Geometry: final body of the model. Coordinates: model frame, mm. A direction names the side the tool comes from. Round coordinates to 2 decimals unless told otherwise and drop trailing zeros. Order: outer loops, then holes, each group sorted by start corner. A loop starts at its lowest first (then second) coordinate and runs counter-clockwise, first axis right, second up. Notation, with made-up numbers: M 45,33.5 L 67,33.5 A15 ccw 67,62.5 Z; hole C 73.5,-35.75 d3. An arc over 180 degrees is marked long. Put each result on its own line as item: value. Start each with the question number.
1) Access query for faces 1 (the flat face through (-8.38, 15.21, 34.31)), 2 (the flat face through (35.002, 15.21, 4.747)), 3 (the flat face through (-31.107, 15.21, 16.734)), 4 (the flat face through (-21.61, 15.21, 27.94)), 5 (the flat face through (6.22, 15.21, -34.64)). Directions: +Z, -Z, +X, -X, +Y, -Y. A direction counts if a zero-diameter tool reaches every point of the face in a straight line with its end or side. Return the directions, or none.
2) First-contact query: P1, Ø1.5, axis at x = 13.5, y = 11, coming from the +Z side; P2, Ø5, axis at x = -3, z = -16, coming from the +Y side; P3, Ø3, axis at y = 9.5, z = 29.5, coming from the +X side; P4, Ø3, axis at y = 22, z = 22.5, coming from the -X side. Flat tips, straight axial feed; report the tip coordinate or a pass-through.
3) Section B-B, the plane z = -10. Return loops of the section in (x, y), then the cut area to 3 significant figures.
4) Draft query along Z for faces 6 (the flat face through (8.5, 0, 18.3)), 7 (the cylindrical face through (26.73, 15.21, 29.76)), 8 (the flat face through (-13.39, 15.21, -32.686)), 9 (the flat face through (33.907, 15.21, -9.9)). Return one class per face: pulls with the +Z half, pulls with the -Z half, needs draft (parallel to the pull), parting line crosses it, or undercut.
5) Section C-C, the plane x = -24.5. Return loops of the section in (y, z), then the cut area to 3 significant figures.
6) Material intervals for probe 1 along Z at (x, y) = (28, 8.5); probe 2 along Z at (x, y) = (28.5, 2.5); probe 3 along Z at (x, y) = (-33.5, 25.5), sorted ascending. Write a range as [from, to].
7) Section A-A, the plane x = 6. Return loops of the section in (y, z).
from build123d import *

# Parameters (mm, degrees)
SKETCH_2_W               = 20
SKETCH_2_H               = 30
CUT_EXTRUDE_1_DEPTH      = 65.031242374
PATTERN_CIRCULAR_2_COUNT = 15


with BuildPart() as part:
    # 草图2 → 旋转1 (revolve)
    with BuildSketch(Plane.XY, mode=Mode.PRIVATE) as revolve_1_sk:
        with Locations((-30, 15)):
            Rectangle(SKETCH_2_W, SKETCH_2_H)
    revolve(revolve_1_sk.sketch.rotate(Axis((0, 0, 0), (0, 1, 0)), 270), axis=Axis((0, 0, 0), (0, 1, 0)))

    # 草图3 → 切除-拉伸1 (cut, through all)
    with BuildSketch(Plane(origin=(0, 30, 0), x_dir=(1, 0, 0), z_dir=(0, 1, 0))):
        Polygon((-30.66106403, 0), (-39.66106403, 5.196152423), (-48.66106403, 0), (-39.66106403, -5.196152423), align=None)
    cut_extrude_1 = extrude(amount=-CUT_EXTRUDE_1_DEPTH, mode=Mode.SUBTRACT)

    # 阵列(圆周)2: 切除-拉伸1 ×15 about axis
    pattern_circular_2_axis = Axis((0, 0, 0), (0, 1, 0))
    for i in range(1, PATTERN_CIRCULAR_2_COUNT):
        add(cut_extrude_1.rotate(pattern_circular_2_axis, i * 360 / PATTERN_CIRCULAR_2_COUNT), mode=Mode.SUBTRACT)


solid = part.part
Result sheet:
1. face 1: +Z, +Y, -Y
1. face 2: +X, +Y, -Y
1. face 3: -X, +Y, -Y
1. face 4: +Y, -Y
1. face 5: -Z, +Y, -Y
2. P1: stops at z = 37.91
2. P2: passes through
2. P3: stops at x = 28.57
2. P4: stops at x = -34.04
3. outline: M -38.73,0 L -17.32,0 L -17.32,30 L -38.73,30 Z; M 17.32,0 L 34.02,0 L 34.02,30 L 17.32,30 Z
3. area: 1,140 mm2
4. face 6: needs draft
4. face 7: pulls with the +Z half
4. face 8: pulls with the -Z half
4. face 9: undercut
5. outline: M 0,-24.08 L 30,-24.08 L 30,24.08 L 0,24.08 Z
5. area: 1,440 mm2
6. probe 1: z = [-28.57, -25.2], [-18.36, 18.36], [25.2, 28.57]
6. probe 2: z = [-28.07, -26.32], [-18.41, 18.41], [26.32, 28.07]
6. probe 3: z = [-21.86, -20.03], [-11.89, -1.64], [1.64, 11.89], [20.03, 21.86]
7. outline: M 0,-34.34 L 30,-34.34 L 30,-19.08 L 0,-19.08 Z; M 0,19.08 L 30,19.08 L 30,34.34 L 0,34.34 Z
